Source: CAD feature listing. Evaluate the final solid. Frame: model axes, mm. A direction names the side the tool comes from. Give positions to 0.01 mm unless a question says otherwise; leave off trailing zeros. Order: outer loops, then holes, each group sorted by start corner. A loop starts at its lowest first (then second) coordinate and runs counter-clockwise, first axis right, second up. Notation, with made-up numbers: (17.25, -8) -> (62.25, -8) arc R22 cw to (62.25, 29) -> close; hole circle Ø4 at (35.5, -34). An arc over 180 degrees is marked (long way). Use one line per item in the form item = value. Start each with the question number.
from build123d import *

# Parameters (mm, degrees)
BOSS_EXTRUDE1_DEPTH = 6.35


with BuildPart() as part:
    # Sketch1 → Boss-Extrude1 (new body)
    with BuildSketch(Plane.XY):
        with BuildLine():
            Line((-11.1506, 0), (11.1506, 0))
            Line((11.1506, 0), (11.1506, -3.81))
            Line((11.1506, -3.81), (17.5006, -3.81))
            Line((17.5006, -3.81), (17.5006, 0))
            Line((17.5006, 0), (17.5006, 6.35))
            Line((17.5006, 6.35), (21.3106, 6.35))
            ThreePointArc((21.3106, 6.35), (23.106651224, 5.606051224), (23.8506, 3.81))
            Line((23.8506, 3.81), (23.8506, -7.62))
            Line((23.8506, -7.62), (23.8506, -13.97))
            Line((23.8506, -13.97), (11.1506, -13.97))
            Line((11.1506, -13.97), (11.1506, -7.62))
            Line((11.1506, -7.62), (-11.1506, -7.62))
            Line((-11.1506, -7.62), (-11.1506, -13.97))
            Line((-11.1506, -13.97), (-23.8506, -13.97))
            Line((-23.8506, -13.97), (-23.8506, -7.62))
            Line((-23.8506, -7.62), (-23.8506, 3.81))
            ThreePointArc((-23.8506, 3.81), (-23.106651224, 5.606051224), (-21.3106, 6.35))
            Line((-21.3106, 6.35), (-17.5006, 6.35))
            Line((-17.5006, 6.35), (-17.5006, 0))
            Line((-17.5006, 0), (-17.5006, -3.81))
            Line((-17.5006, -3.81), (-11.1506, -3.81))
            Line((-11.1506, -3.81), (-11.1506, 0))
        make_face()
    extrude(amount=BOSS_EXTRUDE1_DEPTH)


solid = part.part
1) Draft query along X for faces 1 (the face through (-17, -13.97, 3)), 2 (the face through (23.087, 5.626, 3.131)), 3 (the face through (11.151, -2, 3)). Return one class per face: +X half, -X half, draft (parallel to the pull), parting line (faces both ways), or undercut.
2) Cut plane D-D, the plane x = 17. Return the cut outline in (y, z), plus the area to 3 significant figures.
3) Reachability of faces 4 (the face through (0, -4, 6.35)), 5 (the face through (11.151, -11, 3)), 6 (the face through (0, 0, 3)) from +Z, -Z, +X, -X, +Y, -Y: full face, straight path, thin tool, end or side. Return the list, or none.
4) Cut plane B-B, the plane y = -8.5. Return the cut outline in (x, z).
5) Cut plane C-C, the plane z = 2.5. Return the cut outline in (x, y), plus the area to 3 significant figures.
6) Pin query (flat end, axial travel): pin 1 (1.9 mm diameter, centred on x = 5, z = 2, fed in from -Y); pin 2 (1.9 mm diameter, centred on x = 13.5, z = 4, fed in from +Y). Return the tip coordinate at first contact, or that it passes through.
7) Cut plane A-A, the plane y = -0.5. Return the cut outline in (x, z), plus the area to 3 significant figures.
8) Material intervals for probe 1 along X at (y, z) = (-3, 6.25); probe 2 along X at (y, z) = (-9.5, 5.25); probe 3 along X at (y, z) = (0.5, 4.25), sorted ascending.
Output values:
q1.face_1 = draft
q1.face_2 = +X half
q1.face_3 = undercut
q2.outline = (-13.97, 0) -> (-3.81, 0) -> (-3.81, 6.35) -> (-13.97, 6.35) -> close
q2.area = 64.5 mm^2
q3.face_4 = +Z, +X, -X, +Y, -Y
q3.face_5 = +Z, -Z, -Y
q3.face_6 = +Z, -Z, +Y
q4.outline = (-23.85, 0) -> (-11.15, 0) -> (-11.15, 6.35) -> (-23.85, 6.35) -> close; (11.15, 0) -> (23.85, 0) -> (23.85, 6.35) -> (11.15, 6.35) -> close
q5.outline = (-23.85, -13.97) -> (-11.15, -13.97) -> (-11.15, -7.62) -> (11.15, -7.62) -> (11.15, -13.97) -> (23.85, -13.97) -> (23.85, 3.81) arc R2.54 ccw to (21.31, 6.35) -> (17.5, 6.35) -> (17.5, -3.81) -> (11.15, -3.81) -> (11.15, 0) -> (-11.15, 0) -> (-11.15, -3.81) -> (-17.5, -3.81) -> (-17.5, 6.35) -> (-21.31, 6.35) arc R2.54 ccw to (-23.85, 3.81) -> close
q5.area = 554 mm^2
q6.pin_1 = -7.62
q6.pin_2 = -3.81
q7.outline = (-23.85, 0) -> (-17.5, 0) -> (-17.5, 6.35) -> (-23.85, 6.35) -> close; (-11.15, 0) -> (11.15, 0) -> (11.15, 6.35) -> (-11.15, 6.35) -> close; (17.5, 0) -> (23.85, 0) -> (23.85, 6.35) -> (17.5, 6.35) -> close
q7.area = 222 mm^2
q8.probe_1 = -23.85 to -17.5, -11.15 to 11.15, 17.5 to 23.85
q8.probe_2 = -23.85 to -11.15, 11.15 to 23.85
q8.probe_3 = -23.85 to -17.5, 17.5 to 23.85
